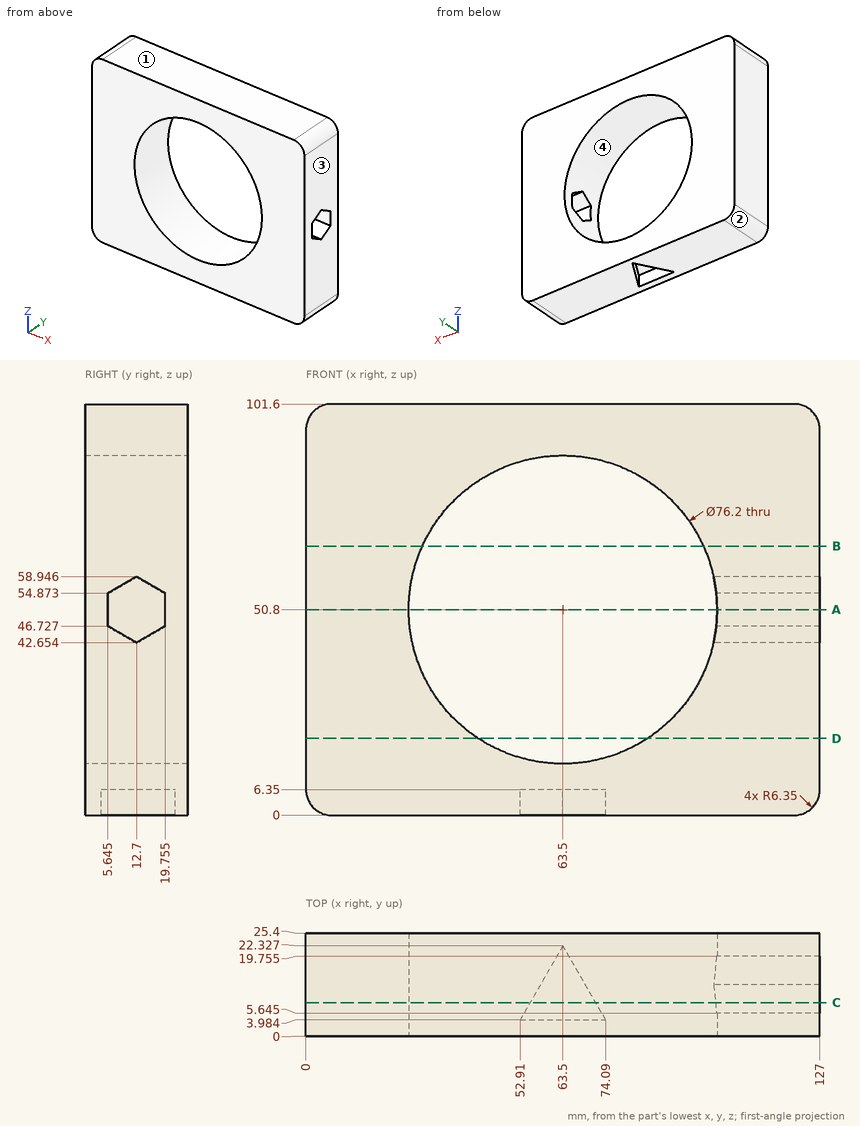
Geometry check sheet. Reference: drawing and pictorial views, mm from the part's lowest x, y, z. Give positions to 0.01 mm unless a question says otherwise; leave off trailing zeros. Order: outer loops, then holes, each group sorted by start corner. A loop starts at its lowest first (then second) coordinate and runs counter-clockwise, first axis right, second up. Notation, with made-up numbers: M -32.75,-29.75 L 0.25,-29.75 A24 cw 0.25,2.25 Z; hole C -21,85 d1. An arc over 180 degrees is marked long. Answer in a Markdown table with one row per item. Add a question column.
Q1. Sectioned sample at B-B, the plane z = 66.5. Record the boundary of the cut face in (x, y) (1 decimal), and give its area (3 significant figures).
Q2. Sectioned sample at C-C, the plane y = 8.25. Record the boundary of the cut face in (x, z), and give its area (3 significant figures).
Q3. Thickness scan on L1, parallel to Y at x = 103, z = 47 (1 decimal); L2, parallel to X at y = 8.5, z = 50.8; L3, parallel to X at y = 5.5, z = 36. Record the ranges inside material, lowest first.
Q4. Sectioned sample at D-D, the plane z = 19. Record the boundary of the cut face in (x, y) (1 decimal), and give its area (3 significant figures).
Q5. Release check for a two-part mould opening along Z. For the marked faces 1, 2, 3 and 4 record: released by +Z, released by -Z, zero draft, split by the parting line, or undercut.
Q6. Sectioned sample at A-A, the plane z = 50.8. Record the boundary of the cut face in (x, y) (1 decimal).
Verdict:
| question | item | result |
|---|---|---|
| 1 | outline | M 0,0 L 28.8,0 L 28.8,25.4 L 0,25.4 Z; M 98.2,0 L 127,0 L 127,25.4 L 98.2,25.4 Z |
| 1 | area | 1,460 mm² |
| 2 | outline | M 0,6.35 A6.35 ccw 6.35,0 L 55.37,0 L 55.37,6.35 L 71.63,6.35 L 71.63,0 L 120.65,0 A6.35 ccw 127,6.35 L 127,45.22 L 101.19,45.22 A38.1 cw long 101.19,56.38 L 127,56.38 L 127,95.25 A6.35 ccw 120.65,101.6 L 6.35,101.6 A6.35 ccw 0,95.25 Z |
| 2 | area | 7,920 mm² |
| 3 | L1 | 0 to 5.6, 19.8 to 25.4 |
| 3 | L2 | 0 to 25.4 |
| 3 | L3 | 0 to 28.39, 98.61 to 127 |
| 4 | outline | M 0,0 L 42.5,0 L 42.5,25.4 L 0,25.4 Z; M 84.5,0 L 127,0 L 127,25.4 L 84.5,25.4 Z |
| 4 | area | 2,160 mm² |
| 5 | face 1 | released by +Z |
| 5 | face 2 | released by -Z |
| 5 | face 3 | zero draft |
| 5 | face 4 | undercut |
| 6 | outline | M 0,0 L 25.4,0 L 25.4,25.4 L 0,25.4 Z; M 101.6,0 L 127,0 L 127,5.6 L 101.6,5.6 Z; M 101.6,19.8 L 127,19.8 L 127,25.4 L 101.6,25.4 Z |
